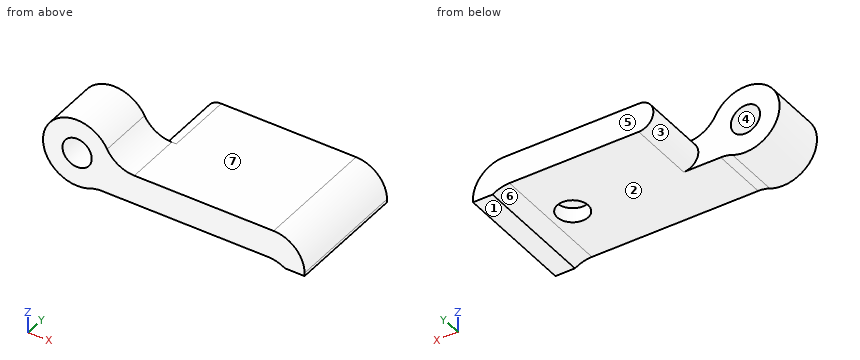
```python
from build123d import *

# Parameters (mm, degrees)
SKETCH1_R           = 3.5
BOSS_EXTRUDE1_DEPTH = 12.7
CUT_EXTRUDE1_START  = -6.93
CUT_EXTRUDE1_DEPTH  = 6.93
SKETCH3_R           = 1.5
CUT_EXTRUDE2_DEPTH  = 6.77
SKETCH4_W           = 2
SKETCH4_H           = 0.5
BOSS_EXTRUDE2_DEPTH = 12.7
FILLET1_R           = 3.175
SKETCH5_R           = 2
CUT_EXTRUDE3_DEPTH  = 10
SKETCH6_R           = 1.585
CUT_EXTRUDE4_DEPTH  = 1.5


with BuildPart() as part:
    # Sketch1 → Boss-Extrude1 (new body)
    with BuildSketch(Plane(origin=(0, 0, 0), x_dir=(1, 0, 0), z_dir=(0, 1, 0))):
        with Locations((-22.063770306, 11.23554707)):
            Circle(SKETCH1_R)
        with BuildLine():
            ThreePointArc((-20.260994668, 14.23554707), (-19.017484475, 12.958957246), (-18.563770306, 11.23554707))
            Line((-18.563770306, 11.23554707), (1.266442488, 11.23554707))
            Line((1.266442488, 11.23554707), (1.266442488, 14.23554707))
            Line((1.266442488, 14.23554707), (-20.260994668, 14.23554707))
        make_face()
    extrude(amount=BOSS_EXTRUDE1_DEPTH)

    # Sketch2 → Cut-Extrude1 (cut)
    with BuildSketch(Plane(origin=(0, 12.7, 0), x_dir=(1, 0, 0), z_dir=(0, 1, 0)).offset(CUT_EXTRUDE1_START)):
        with BuildLine():
            Line((-18.563770306, 11.23554707), (-15.733557512, 11.23554707))
            ThreePointArc((-15.733557512, 11.23554707), (-17.233557512, 12.73554707), (-15.733557512, 14.23554707))
            Line((-15.733557512, 14.23554707), (-20.260994668, 14.23554707))
            ThreePointArc((-20.260994668, 14.23554707), (-25.110056137, 9.512136894), (-18.563770306, 11.23554707))
        make_face()
    extrude(amount=CUT_EXTRUDE1_DEPTH, mode=Mode.SUBTRACT)

    # Sketch3 → Cut-Extrude2 (cut, through all)
    with BuildSketch(Plane(origin=(0, 5.77, 0), x_dir=(1, 0, 0), z_dir=(0, 1, 0))):
        with Locations(Location((-22.063770306, 11.23554707, 0), (0, 0, 270))):  # turned: the seam where the file's is
            Circle(SKETCH3_R)
    extrude(amount=-CUT_EXTRUDE2_DEPTH, mode=Mode.SUBTRACT)

    # Sketch4 → Boss-Extrude2 (add)
    with BuildSketch(Plane(origin=(0, 12.7, 0), x_dir=(1, 0, 0), z_dir=(0, 1, 0))):
        with Locations((0.266442488, 14.48554707)):
            Rectangle(SKETCH4_W, SKETCH4_H)
        with BuildLine():
            Line((-2.472810226, 14.23554707), (-0.733557512, 14.23554707))
            Line((-0.733557512, 14.23554707), (-0.733557512, 14.73554707))
            ThreePointArc((-0.733557512, 14.73554707), (-1.567962172, 14.363028206), (-2.472810226, 14.23554707))
        make_face()
    extrude(amount=-BOSS_EXTRUDE2_DEPTH)

    # Fillet1
    fillet1_edges = [part.edges().sort_by_distance(p)[0] for p in [
        (-20.260994668, 2.885, -14.23554707),
        (-18.563770306, 2.885, -11.23554707),
        (1.266442488, 6.35, -11.23554707),
    ]]
    fillet(fillet1_edges, radius=FILLET1_R)

    # Sketch5 → Cut-Extrude3 (cut)
    with BuildSketch(Plane(origin=(0, 0, -14.23554707), x_dir=(-1, 0, 0), z_dir=(0, 0, -1))):
        with Locations((-37.221491695, -42.831378851)):
            Circle(SKETCH5_R)
        with Locations((-37.221491695, -47.531378851)):
            Circle(SKETCH5_R)
    extrude(amount=-CUT_EXTRUDE3_DEPTH, mode=Mode.SUBTRACT)

    # Sketch6 → Cut-Extrude4 (cut)
    with BuildSketch(Plane(origin=(0, 0, -14.23554707), x_dir=(-1, 0, 0), z_dir=(0, 0, -1))):
        with Locations((4.733557512, 6.35)):
            Circle(SKETCH6_R)
    extrude(amount=-CUT_EXTRUDE4_DEPTH, mode=Mode.SUBTRACT)


solid = part.part
```
Read the model definition and answer for the solid it produces. Units are mm, in the model's axes. Face numbers are marked on the shaded views. A direction names the side the tool comes from. Give positions to 0.01 mm unless a question says otherwise; leave off trailing zeros. Order: outer loops, then holes, each group sorted by start corner. A loop starts at its lowest first (then second) coordinate and runs counter-clockwise, first axis right, second up. Notation, with made-up numbers: (43.25, -4) -> (100.25, -4) arc R22 ccw to (100.25, 14) -> close; hole circle Ø2 at (4.5, 9). An arc over 180 degrees is marked (long way). Write item = value, one per line.
1. A cutting plane is placed at C-C, the plane y = 6.35. Write down the section's boundary in (x, z) (3 decimals), and give its area (3 significant figures).
Numbers:
outline = (-15.734, -14.236) -> (-6.319, -14.236) -> (-6.319, -12.736) -> (-3.149, -12.736) -> (-3.149, -14.236) -> (-2.473, -14.236) arc R3.275 cw to (-0.734, -14.736) -> (1.266, -14.736) -> (1.266, -14.411) arc R3.175 ccw to (-1.909, -11.236) -> (-15.734, -11.236) arc R1.5 ccw to start
area = 48.9 mm²
2. A cutting plane is placed at D-D, the plane x = -3.5. Write down the section's boundary in (y, z), and give its area (3 significant figures).
Numbers:
outline = (0, -14.24) -> (5.35, -14.24) -> (5.35, -12.74) -> (7.35, -12.74) -> (7.35, -14.24) -> (12.7, -14.24) -> (12.7, -11.24) -> (0, -11.24) -> close
area = 35.1 mm²
3. The mould has two halves that part along X. Classify the marked faces 1, 2, 3 and 4: +X half, -X half, draft (parallel to the pull), parting line (faces both ways), or undercut.
Numbers:
face_1 = draft
face_2 = undercut
face_3 = -X half
face_4 = undercut
4. Straight lines are drawn through the part: line 1 along Z through (x, y) = (-4, 9); line 2 along Y through (x, z) = (-17.75, -12.5); line 3 along X through (y, z) = (1.25, -12.25). For each, find the intervals that lie inside material, in ascending order.
Numbers:
line_1 = -14.24 to -11.24
line_2 = 0 to 5.77
line_3 = -25.41 to -23.17, -20.96 to 0.42
5. A cutting plane is placed at A-A, the plane z = -10.25. Write down the section's boundary in (x, y), and give its area (3 significant figures).
Numbers:
outline = (-25.42, 0) -> (-23.19, 0) -> (-23.19, 5.77) -> (-25.42, 5.77) -> close; (-20.93, 0) -> (-18.49, 0) -> (-18.49, 5.77) -> (-20.93, 5.77) -> close
area = 26.9 mm²
6. For the marked faces 5, 6 and 7, determine the directions among +Z, -Z, +X, -X, +Y, -Y from which every point of the face is accessible in a straight line to the end or side of a thin tool.
Numbers:
face_5 = +Z, -Z, +X, -X, +Y
face_6 = -Z, +Y, -Y
face_7 = +Z, +X, +Y, -Y
7. A cutting plane is placed at B-B, the plane y = 4. Write down the section's boundary in (x, z) (3 decimals).
Numbers:
outline = (-20.735, -14.473) arc R3.175 cw to (-19.529, -14.236) -> (-2.473, -14.236) arc R3.275 cw to (-0.734, -14.736) -> (1.266, -14.736) -> (1.266, -14.411) arc R3.175 ccw to (-1.909, -11.236) -> (-16.192, -11.236) arc R3.175 cw to (-18.985, -9.571) arc R3.5 ccw (long way) to start; hole circle Ø3 at (-22.064, -11.236)
8. Given pin 1 (4 mm diameter, centred on x = -22.5, z = -14, fed in from +Y); pin 2 (4 mm diameter, centred on x = -9.5, y = 7, fed in from -Z); pin 3 (3 mm diameter, centred on y = 7, z = -12, fed in from -X); pin 4 (1.9 mm diameter, centred on x = -4.73, y = 6.35, fed in from +Z), each flat-ended and moving along its own axis, determine where each tip first touches the part or whether it passes through.
Numbers:
pin_1 = 5.77
pin_2 = -14.24
pin_3 = -25.56
pin_4 = -11.24
